```python
from build123d import *

# Parameters (mm, degrees)
CUT_EXTRUDE3_DEPTH = 0.254
CIRPATTERN1_COUNT  = 6
CUT_EXTRUDE4_DEPTH = 0.254
CIRPATTERN2_COUNT  = 6


with BuildPart() as part:
    # Sketch2 → Revolve1 (revolve)
    with BuildSketch(Plane(origin=(0, 0, 0), x_dir=(1, 0, 0), z_dir=(0, 1, 0))):
        Polygon((4.445, -9.017), (5.842, -6.58754254), (5.842, -6.33354254), (4.826, -6.33354254), (4.826, -4.30154254), (5.842, -4.30154254), (3.967830419, 9.017), (1.5875, 9.017), (1.5875, -9.017), align=None)
    revolve(axis=Axis((0, 0, -9.017), (0, 0, 1)))

    # Sketch3 → Cut-Extrude3 (cut, symmetric)
    with BuildSketch(Plane(origin=(0, 0, 0), x_dir=(0, 0, -1), z_dir=(1, 0, 0))):
        Polygon((-7.605911738, 5.256411738), (-7.605911738, 26.9875), (9.017, 26.9875), (9.017, 0.3175), (-2.667, 0.3175), align=None)
    cut_extrude3 = extrude(amount=CUT_EXTRUDE3_DEPTH, both=True, mode=Mode.SUBTRACT)

    # CirPattern1: Cut-Extrude3 ×6 about axis
    cirpattern1_axis = Axis((0, 0, 0), (0, 0, 1))
    for i in range(1, CIRPATTERN1_COUNT):
        add(cut_extrude3.rotate(cirpattern1_axis, i * 360 / CIRPATTERN1_COUNT), mode=Mode.SUBTRACT)

    # Sketch4 → Cut-Extrude4 (cut, symmetric)
    with BuildSketch(Plane(origin=(0, 0, 0), x_dir=(1, 0, 0), z_dir=(0, 1, 0))):
        Polygon((4.300861057, 6.650361057), (26.9875, 6.650361057), (26.9875, -9.017), (1.5875, -9.017), (0.3175, -9.017), (0.3175, 2.667), align=None)
    cut_extrude4 = extrude(amount=CUT_EXTRUDE4_DEPTH, both=True, mode=Mode.SUBTRACT)

    # CirPattern2: Cut-Extrude4 ×6 about axis
    cirpattern2_axis = Axis((0, 0, 0), (0, 0, 1))
    for i in range(1, CIRPATTERN2_COUNT):
        add(cut_extrude4.rotate(cirpattern2_axis, i * 360 / CIRPATTERN2_COUNT), mode=Mode.SUBTRACT)


solid = part.part
```
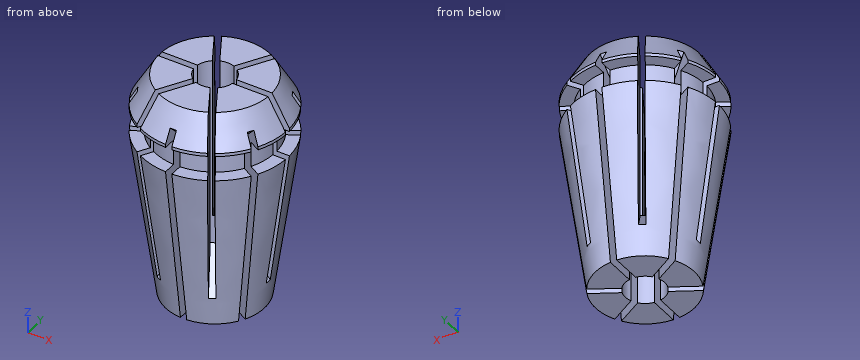
Geometry check sheet. Reference: the model listing, model coordinates, mm. Coordinates: 2 decimals unless noted, no trailing zeros. Write each loop counter-clockwise with the first axis right and the second up, starting at its lowest first coordinate (ties: lowest second). Pieces come first, ordered by that corner, then holes. Notation, with made-up numbers: (83.25, 26) -> (112.25, 26) arc R37 cw to (112.25, 65) -> close; hole circle Ø1 at (-2, -27.75). An arc over 180 degrees is marked (long way). Use CSV: the item, a comma, the result in double quotes. Start each with the question number.
Item 1: Thickness scan on line 1 (X direction, y = 4, z = 3.75); line 2 (X direction, y = 2, z = 5); line 3 (X direction, y = 2.5, z = -0.5). Record the ranges inside material, lowest first.
Item 2: Cross-section at A-A, the plane y = 0. Record the cut outline in (x, z), plus the area to 3 significant figures.
Item 3: Depth check by flat-ended pin: pin 1 Ø3 at (x, y) = (0, -1) entering from -Z; pin 2 Ø5 at (y, z) = (-3, -0.5) entering from -X; pin 3 Ø1.3 at (y, z) = (3.5, 3.5) entering from +X; pin 4 Ø0.8 at (x, y) = (5, 1.5) entering from +Z. Enter the tip coordinate at first touch or a pass-through.
Item 4: Cross-section at B-B, the plane z = -7.5. Record the cut outline in (x, y) (1 decimal).
Item 5: Cross-section at C-C, the plane z = 0.75. State how many separate pieces and enclosed holes the cut face has, plus the area to 3 significant figures.
Answers:
1,line 1,"-4.15 to -2.6, -2.02 to -0.25, 0.25 to 2.02, 2.6 to 4.15"
1,line 2,"-4.39 to -3.97, -2.96 to -1.45, -0.86 to 0.86, 1.45 to 2.96, 3.97 to 4.39"
1,line 3,"-3.82 to -1.74, -1.15 to -0.25, 0.25 to 1.15, 1.74 to 3.82"
2,outline,"(-4.3, -6.65) -> (-3.97, -9.02) -> (-1.59, -9.02) -> (-1.59, -3.94) -> close; (1.59, -9.02) -> (3.97, -9.02) -> (4.3, -6.65) -> (1.59, -3.94) -> close"
2,area,"19.4 mm^2"
3,pin 1,"z = -9.02"
3,pin 2,"x = -5.28"
3,pin 3,"x = 4.89"
3,pin 4,"z = 8.36"
4,outline,"(-3.7, -1.9) -> (-1.5, -0.6) arc R1.6 cw to (-1.5, 0.6) -> (-3.7, 1.9) arc R4.2 ccw to start; (-3.5, -2.3) arc R4.2 ccw to (-0.3, -4.2) -> (-0.3, -1.6) arc R1.6 cw to (-1.2, -1) -> close; (-3.5, 2.3) -> (-1.2, 1) arc R1.6 cw to (-0.3, 1.6) -> (-0.3, 4.2) arc R4.2 ccw to start; (0.3, -4.2) arc R4.2 ccw to (3.5, -2.3) -> (1.2, -1) arc R1.6 cw to (0.3, -1.6) -> close; (0.3, 1.6) arc R1.6 cw to (1.2, 1) -> (3.5, 2.3) arc R4.2 ccw to (0.3, 4.2) -> close; (1.5, -0.6) -> (3.7, -1.9) arc R4.2 ccw to (3.7, 1.9) -> (1.5, 0.6) arc R1.6 cw to start"
5,separate pieces,"12"
5,enclosed holes,"0"
5,area,"58.8 mm^2"
